Work out the finished part from the listing and answer in its coordinate system (mm). Round coordinates to 2 decimals unless told otherwise and drop trailing zeros. Loops run counter-clockwise (first coordinate to the right, second up) from the corner with the lowest first, then second, coordinate; pieces in that order, holes last.
```python
from build123d import *

# Parameters (mm, degrees)
MODEL_R         = 10
MODEL_W         = 4.4
MODEL_H         = 10
EXTRUDE_1_DEPTH = 2


with BuildPart() as part:
    # Model → 凸台-拉伸1 (new body)
    with BuildSketch(Plane.XY):
        Polygon((13.943428414, 55.11082042), (18.943428414, 55.11082042), (18.943428414, 56.11082042), (48.943428414, 56.11082042), (48.943428414, 55.11082042), (108.943428414, 55.11082042), (108.943428414, 56.11082042), (138.943428414, 56.11082042), (138.943428414, 55.11082042), (168.943428414, 55.11082042), (168.943428414, 45.11082042), (166.743428414, 45.11082042), (166.743428414, 35.11082042), (168.943428414, 35.11082042), (168.943428414, 25.11082042), (166.743428414, 25.11082042), (166.743428414, 15.11082042), (168.943428414, 15.11082042), (168.943428414, 5.11082042), (138.943428414, 5.11082042), (138.943428414, 4.11082042), (108.943428414, 4.11082042), (108.943428414, 5.11082042), (61.943428414, 5.11082042), (55.943428414, 5.11082042), (48.943428414, 5.11082042), (48.943428414, 4.11082042), (18.943428414, 4.11082042), (18.943428414, 5.11082042), (6.91562917, 5.11082042), (6.91562917, 55.11082042), align=None)
        with Locations((75.843428414, 30.11082042)):
            Circle(MODEL_R, mode=Mode.SUBTRACT)
        with Locations((106.843428414, 30.11082042)):
            Circle(MODEL_R, mode=Mode.SUBTRACT)
        Polygon((89.690784519, 25.117395738), (91.890784519, 25.108786537), (91.89091955, 15.117786537), (89.690784519, 15.117786537), align=None, mode=Mode.SUBTRACT)
        Polygon((89.690784519, 45.110819609), (91.890784519, 45.102210408), (91.890784519, 35.110819609), (89.690784519, 35.110819609), align=None, mode=Mode.SUBTRACT)
        Polygon((121.843427205, 45.110819609), (124.143292174, 45.101819609), (124.143427205, 35.110819609), (121.843427205, 35.110819609), align=None, mode=Mode.SUBTRACT)
        Polygon((121.843427205, 25.110819609), (124.143292174, 25.101819609), (124.143427205, 15.110819609), (121.843427205, 15.110819609), align=None, mode=Mode.SUBTRACT)
        Polygon((57.844211187, 45.110819609), (60.044211187, 45.11081939), (60.044211187, 35.110819675), (57.844211187, 35.1108198), align=None, mode=Mode.SUBTRACT)
        Polygon((57.844211187, 25.110819609), (60.044211187, 25.11081939), (60.044211187, 15.110819675), (57.844211187, 15.1108198), align=None, mode=Mode.SUBTRACT)
        with Locations((14.11562917, 40.110820275)):
            Rectangle(MODEL_W, MODEL_H, mode=Mode.SUBTRACT)
        with Locations((14.11562917, 20.110820275)):
            Rectangle(MODEL_W, MODEL_H, mode=Mode.SUBTRACT)
    extrude(amount=EXTRUDE_1_DEPTH)


solid = part.part
```
1. Find section A-A (x = 71). Write down the section's boundary in (y, z).
Answer key:
outline: (5.11, 0) - (21.36, 0) - (21.36, 2) - (5.11, 2) - close; (38.86, 0) - (55.11, 0) - (55.11, 2) - (38.86, 2) - close
2. Consider probe 1 along X at (y, z) = (43, 1.45); probe 2 along X at (y, z) = (30, 1.1); probe 3 along X at (y, z) = (31, 1.6). Determine where each line is inside the solid, lowest interval first.
Answer key:
probe 1: x = 6.92 to 11.92, 16.32 to 57.84, 60.04 to 89.69, 91.89 to 121.84, 124.14 to 166.74
probe 2: x = 6.92 to 65.84, 85.84 to 96.84, 116.84 to 168.94
probe 3: x = 6.92 to 65.88, 85.8 to 96.88, 116.8 to 168.94
3. Find section B-B (y = 43). Write down the section's boundary in (x, z).
Answer key:
outline: (6.92, 0) - (11.92, 0) - (11.92, 2) - (6.92, 2) - close; (16.32, 0) - (57.84, 0) - (57.84, 2) - (16.32, 2) - close; (60.04, 0) - (89.69, 0) - (89.69, 2) - (60.04, 2) - close; (91.89, 0) - (121.84, 0) - (121.84, 2) - (91.89, 2) - close; (124.14, 0) - (166.74, 0) - (166.74, 2) - (124.14, 2) - close
4. Find section C-C (y = 22). Write down the section's boundary in (x, z), then the cut area to 3 significant figures.
Answer key:
outline: (6.92, 0) - (11.92, 0) - (11.92, 2) - (6.92, 2) - close; (16.32, 0) - (57.84, 0) - (57.84, 2) - (16.32, 2) - close; (60.04, 0) - (69.99, 0) - (69.99, 2) - (60.04, 2) - close; (81.69, 0) - (89.69, 0) - (89.69, 2) - (81.69, 2) - close; (91.89, 0) - (100.99, 0) - (100.99, 2) - (91.89, 2) - close; (112.69, 0) - (121.84, 0) - (121.84, 2) - (112.69, 2) - close; (124.14, 0) - (166.74, 0) - (166.74, 2) - (124.14, 2) - close
area: 251 mm2
5. Determine the mould class of faces 1 (the face through (89, 30, 0)), 2 (the face through (111.46, 21.24, 0.99)) for opening direction X: +X half, -X half, draft (parallel to the pull), parting line (faces both ways), or undercut.
Answer key:
face 1: draft
face 2: undercut
6. Given pin 1 (12 mm diameter, centred on x = 75.84, y = 30.11, fed in from -Z); pin 2 (1 mm diameter, centred on x = 146.5, z = 1, fed in from -Y); pin 3 (0.5 mm diameter, centred on y = 4.5, z = 1, fed in from +X), each flat-ended and moving along its own axis, determine where each tip first touches the part or whether it passes through.
Answer key:
pin 1: passes through
pin 2: stops at y = 5.11
pin 3: stops at x = 138.94
7. Find section D-D (z = 1.3). Give the number of separate pieces and of enclosed holes in the cut face, then the cut area to 3 significant figures.
Answer key:
separate pieces: 1
enclosed holes: 10
area: 7,330 mm2
